Model file for the job. Use its own axes, mm. Face numbers are marked on the shaded views. A direction names the side the tool comes from. Round coordinates to 2 decimals unless told otherwise and drop trailing zeros. Order: outer loops, then holes, each group sorted by start corner. A loop starts at its lowest first (then second) coordinate and runs counter-clockwise, first axis right, second up. Notation, with made-up numbers: M -10.5,-16 L 8.5,-16 A14 ccw 8.5,4 Z; hole C 44,-11.5 d1. An arc over 180 degrees is marked long. Return JSON: item names as keys, results as strings. Group by question number.
Item 1: Slice it at D-D on y = 4. Write the cut outline in (x, z).
Item 2: Pull direction X, two halves, no side cores. Call the marked faces 4, 5, 6 and 7: pulls with the +X half, pulls with the -X half, needs draft (parallel to the pull), parting line crosses it, or undercut.
Item 3: Probe line 1 along Z through (x, y) = (0, 60); line 2 along X through (y, z) = (27, 22); line 3 along Y through (x, z) = (-21.5, 35). List the from-to ranges inside material, lowest first.
Item 4: Slice it at A-A on z = 35. Write the cut outline in (x, y).
Item 5: Pin check, flat tips, straight feed: pin 1 Ø16 at (y, z) = (-7.78, 42.88) entering from +X; pin 2 Ø12 at (y, z) = (70, 45) entering from -X; pin 3 Ø1.5 at (x, z) = (-20.5, 45.5) entering from +Y; pin 4 Ø3 at (x, z) = (-30, 44) entering from -Y. Stop position of each tip, or through.
Item 6: Slice it at B-B on z = 14.5. Write the cut outline in (x, y).
Item 7: Slice it at C-C on x = 5. Write the cut outline in (y, z), then the cut area to 3 significant figures.
Item 8: Which spindle directions (+Z, -Z, +X, -X, +Y, -Y) get a long thin tool onto all of the face, cutting with end or side? Do the marked faces 1, 2 and 3. Say none if no direction does.
Autodesk Inventor part; units mm, degrees
ref_plane "YZ Plane" through (0, 0, 0) normal (1, 0, 0) x (0, 1, 0)
ref_plane "XZ Plane" through (0, 0, 0) normal (0, 1, 0) x (-1, 0, 0)
ref_plane "XY Plane" through (0, 0, 0) normal (0, 0, 1) x (1, 0, 0)
sketch "Sketch1" plane through (0, 0, 0) normal (1, 0, 0) x (0, 1, 0)
  line L0 (28.0764, 57.8828) -> (-21.9236, 57.8828)
  line L1 (-21.9236, 57.8828) -> (-21.9236, 7.8828)
  line L2 (-21.9236, 7.8828) -> (28.0764, 7.8828)
  line L3 (28.0764, 7.8828) -> (28.0764, 57.8828)
  circle A0 centre (-7.7792, 22.8828) radius 5
  circle A1 centre (-7.7792, 42.8828) radius 5
  point P0 (0, 0)
  dimension "d0" = 50
  dimension "d1" = 50
  dimension "d3" = 10
  dimension "d5" = 10
extrude "Extrusion1" add sketch "Sketch1" along normal blind 20
sketch "Sketch2" plane through (0, -21.9236, 57.8828) normal (0, 0, 1) x (1, 0, 0)
  line L0 (20, 0) -> (20, 50)
  line L1 (20, 50) -> (-25, 127.9423)
  line L2 (20, 50) -> (110, 50) construction
  line L3 (0, 50) -> (-45, 127.9423)
  line L4 (0, 50) -> (90, 50) construction
  line L5 (-45, 127.9423) -> (-25, 127.9423)
  line L6 (0, 50) -> (20, 50)
  point P0 (0, 21.9236)
  dimension "d8" = 90
  dimension "d9" = 120
  dimension "d10" = 90
  dimension "d11" = 120
extrude "Extrusion2" add sketch "Sketch2" against normal blind 50
sketch "Sketch3" plane through (20, 28.0764, 57.8828) normal (0.866, 0.5, 0) x (0, 0, -1)
  line L0 (0, 0) -> (0, -43.3013)
  line L1 (0, 0) -> (0, 90)
  arc A0 (40, 75) -> (10, 75) centre (25, 75) ccw
  line L2 (0, 0) -> (0, 45)
  line L3 (50, 0) -> (0, 0)
  line L4 (0, 0) -> (50, 0)
  line L5 (50, 0) -> (50, 45)
  arc A1 (5.4018, 67.7593) -> (10, 75) centre (2, 75) ccw
  line L6 (10, 75) -> (2, 75) construction
  line L7 (4.7362, 67.4825) -> (2, 75) construction
  arc A2 (40, 75) -> (44.5982, 67.7593) centre (48, 75) ccw
  line L8 (40, 75) -> (48, 75) construction
  line L9 (45.2638, 67.4825) -> (48, 75) construction
  arc A3 (4.4105, 66.7289) -> (0, 45) centre (55.73, 45) ccw
  arc A4 (50, 45) -> (45.5895, 66.7289) centre (-5.73, 45) ccw
  arc A5 (5.4018, 67.7593) -> (4.4105, 66.7289) centre (6.2523, 65.9491) ccw
  arc A6 (45.5895, 66.7289) -> (44.5982, 67.7593) centre (43.7477, 65.9491) ccw
  line L10 (25, 90) -> (0, 90)
  line L11 (0, 90) -> (0, 45)
  line L12 (50, 90) -> (50, 0)
  line L13 (50, 90) -> (50, 45)
  line L14 (25, 90) -> (50, 90)
  point P0 (57.8828, -14.3149)
  dimension "d18" = 45
  dimension "d19" = 45
  dimension "d20" = 8
  dimension "d21" = 70
  dimension "d22" = 8
  dimension "d23" = 70
  dimension "d24" = 2
  dimension "d25" = 2
extrude "Extrusion3" cut sketch "Sketch3" against normal blind 50 contours L1 L10 A0 A1 A5 A3 | A4 A6 A2 A0 L14 L12
sketch "Sketch4" plane through (-40, 97.3585, 32.8828) normal (0.5, -0.866, 0) x (0.866, 0.5, 0)
  line L0 (17.3205, 25) -> (17.3205, 0)
  line L1 (17.3205, 0) -> (17.3205, -25)
  line L2 (17.3205, 25) -> (17.3205, -25)
  line L3 (17.3205, -25) -> (-0.3461, -25)
  line L4 (-0.3461, -25) -> (-0.3461, 25)
  line L5 (17.3205, 25) -> (0, 25)
  line L6 (-0.3461, 25) -> (17.3205, 25)
  point P0 (-14.0382, -32.8828)
  point P1 (0, 25)
extrude "Extrusion4" cut sketch "Sketch4" against normal blind 50
sketch "Sketch5" plane through (20, 28.0764, 57.8828) normal (0.866, 0.5, 0) x (0, 0, -1)
  line L0 (50, 0) -> (0, 0)
  circle A0 centre (25, 75) radius 5
  point P0 (57.8828, -14.3149)
  dimension "d32" = 10
extrude "Extrusion5" cut sketch "Sketch5" against normal blind 50
sketch "Sketch6" plane through (20, 28.0764, 57.8828) normal (0.866, 0.5, 0) x (0, 0, -1)
  line L0 (0, 0) -> (0, 45)
  line L1 (50, 0) -> (0, 0)
  line L2 (25, 68.094) -> (45, 56.547)
  line L3 (45, 56.547) -> (45, 33.453)
  line L4 (45, 33.453) -> (25, 21.906)
  line L5 (25, 21.906) -> (5, 33.453)
  line L6 (5, 33.453) -> (5, 56.547)
  line L7 (5, 56.547) -> (25, 68.094)
  point P0 (57.8828, -14.3149)
  point P1 (25, 45)
  point P2 (45, 45)
  point P3 (5, 45)
  dimension "d37" = 40
extrude "Extrusion6" cut sketch "Sketch6" against normal blind 30
properties part number "6 - Part  5"
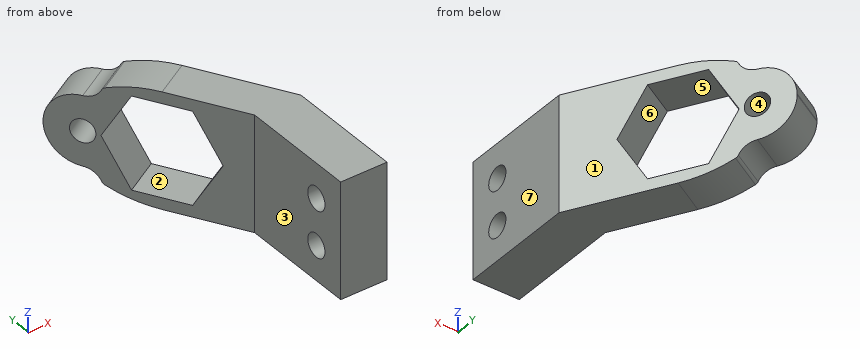
Output values:
{
 "1": {"outline": "M 0,7.88 L 20,7.88 L 20,57.88 L 0,57.88 Z"},
 "2": {"face 4": "undercut", "face 5": "needs draft", "face 6": "pulls with the -X half", "face 7": "pulls with the +X half"},
 "3": {"line 1": "7.88 to 12.88, 52.88 to 57.88", "line 2": "0 to 20", "line 3": "81.33 to 85.49, 95.95 to 99.96"},
 "4": {"outline": "M -39.92,97.23 L -34.76,88.29 L -19.76,96.95 L -24.92,105.89 Z; M -30.24,80.45 L -28.44,77.33 L -13.44,85.99 L -15.24,89.11 Z; M -6.56,39.45 L 0,28.08 L 0,-21.92 L 20,-21.92 L 20,28.08 L 8.44,48.11 Z"},
 "5": {"pin 1": "x = 20", "pin 2": "x = -27.67", "pin 3": "y = 99.52", "pin 4": "y = 77.44"},
 "6": {"outline": "M -29.23,78.71 L -23.74,69.2 L -8.74,77.86 L -14.23,87.37 Z; M -11.26,47.58 L 0,28.08 L 0,-21.92 L 20,-21.92 L 20,28.08 L 3.74,56.24 Z"},
 "7": {"outline": "M -21.92,7.88 L 54.06,7.88 L 54.06,18.86 L 44.71,32.88 L 54.06,46.9 L 54.06,57.88 L -21.92,57.88 Z; hole C -7.78,22.88 d10; hole C -7.78,42.88 d10", "area": "3,510 mm²"},
 "8": {"face 1": "+Z, -Z, +X, +Y", "face 2": "none", "face 3": "+Z, -Z, -X, -Y"}
}
